Check sheet for the modelled part. Datum: model origin and axes. Units: mm. Give positions to 0.01 mm unless a question says otherwise; leave off trailing zeros. Order: outer loops, then holes, each group sorted by start corner. A loop starts at its lowest first (then second) coordinate and runs counter-clockwise, first axis right, second up.
Item 1: Sectioned sample at A-A on x = 0. Record the boundary of the cut face in (y, z).
Item 2: Sectioned sample at C-C on x = 120. Record the boundary of the cut face in (y, z), and give its area (3 significant figures).
Item 3: Material ranges on line 1 along X through (y, z) = (2, 0); line 2 along X through (y, z) = (2.75, -15.5); line 3 along Z through (x, y) = (-15, 3.4), recorded low to high.
Item 4: Gauge pin test, flat ends, axial feed: P1, Ø2, axis at x = 83.5, y = 2, coming from the -Z side; P2, Ø2.5, axis at x = -64.5, y = 1.5, coming from the -Z side; P3, Ø2.5, axis at x = 36.08, z = 62.5, coming from the -Y side; P4, Ø3, axis at y = 2, z = 9, coming from the -X side. Record the tip position at first contact, or that the pin passes through.
Item 5: Sectioned sample at D-D on z = -83.5. Record the boundary of the cut face in (x, y), and give its area (3 significant figures).
Item 6: Sectioned sample at B-B on y = 1.85. Count the separate pieces of the cut face and the enclosed holes in it, and give its area (3 significant figures).
from build123d import *

# Parameters (mm, degrees)
SKETCH_1_R      = 150
SKETCH_1_R_2    = 1.5
SKETCH_1_R_3    = 12.5
SKETCH_1_R_4    = 2
SKETCH_1_W      = 5
SKETCH_1_H      = 4
EXTRUDE_1_DEPTH = 5


with BuildPart() as part:
    # 草图1 → 凸台-拉伸1 (new body)
    with BuildSketch(Plane(origin=(0, 0, 0), x_dir=(1, 0, 0), z_dir=(0, 1, 0))):
        with Locations(Location((0, 0, 0), (0, 0, 270))):
            Circle(SKETCH_1_R)
        with Locations(Location((-15.5, 15.5, 0), (0, 0, 270))):
            Circle(SKETCH_1_R_2, mode=Mode.SUBTRACT)
        with Locations(Location((15.5, 15.5, 0), (0, 0, 270))):
            Circle(SKETCH_1_R_2, mode=Mode.SUBTRACT)
        with Locations(Location((15.5, -15.5, 0), (0, 0, 270))):
            Circle(SKETCH_1_R_2, mode=Mode.SUBTRACT)
        with Locations(Location((-15.5, -15.5, 0), (0, 0, 270))):
            Circle(SKETCH_1_R_2, mode=Mode.SUBTRACT)
        with Locations(Location((0, 0, 0), (0, 0, 270))):
            Circle(SKETCH_1_R_3, mode=Mode.SUBTRACT)
        with Locations(Location((-72.168783649, 0, 0), (0, 0, 270))):
            Circle(SKETCH_1_R_4, mode=Mode.SUBTRACT)
        with Locations(Location((36.084391824, 62.5, 0), (0, 0, 270))):
            Circle(SKETCH_1_R_4, mode=Mode.SUBTRACT)
        with Locations(Location((36.084391824, -62.5, 0), (0, 0, 270))):
            Circle(SKETCH_1_R_4, mode=Mode.SUBTRACT)
        Polygon((36.852341017, 67.830127019), (40.316442632, 65.830127019), (42.816442632, 70.160254038), (39.352341017, 72.160254038), align=None, mode=Mode.SUBTRACT)
        with Locations((-64.668783649, 0)):
            Rectangle(SKETCH_1_W, SKETCH_1_H, mode=Mode.SUBTRACT)
        with Locations((-79.668783649, 0)):
            Rectangle(SKETCH_1_W, SKETCH_1_H, mode=Mode.SUBTRACT)
        Polygon((29.352341017, 54.839745962), (32.816442632, 52.839745962), (35.316442632, 57.169872981), (31.852341017, 59.169872981), align=None, mode=Mode.SUBTRACT)
        Polygon((40.316442632, -65.830127019), (36.852341017, -67.830127019), (39.352341017, -72.160254038), (42.816442632, -70.160254038), align=None, mode=Mode.SUBTRACT)
        Polygon((32.816442632, -52.839745962), (29.352341017, -54.839745962), (31.852341017, -59.169872981), (35.316442632, -57.169872981), align=None, mode=Mode.SUBTRACT)
    extrude(amount=EXTRUDE_1_DEPTH)


solid = part.part
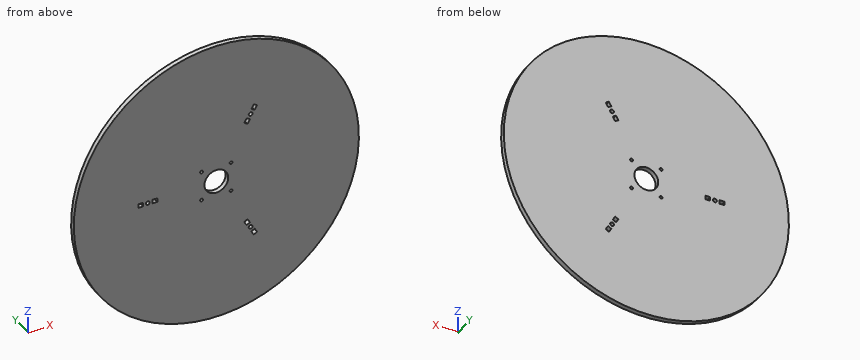
Report:
1. outline: (0, -150) - (5, -150) - (5, -12.5) - (0, -12.5) - close; (0, 12.5) - (5, 12.5) - (5, 150) - (0, 150) - close
2. outline: (0, -90) - (5, -90) - (5, 90) - (0, 90) - close
2. area: 900 mm2
3. line 1: x = -150 to -82.17, -77.17 to -74.17, -70.17 to -67.17, -62.17 to -12.5, 12.5 to 150
3. line 2: x = -149.2 to -17, -14 to 14, 17 to 149.2
3. line 3: z = -149.25 to -16.91, -14.09 to 14.09, 16.91 to 149.25
4. P1: stops at z = -125.27
4. P2: stops at z = -136.01
4. P3: passes through
4. P4: stops at x = -149.81
5. outline: (-124.61, 0) - (124.61, 0) - (124.61, 5) - (-124.61, 5) - close
5. area: 1,250 mm2
6. separate pieces: 1
6. enclosed holes: 14
6. area: 70,000 mm2
